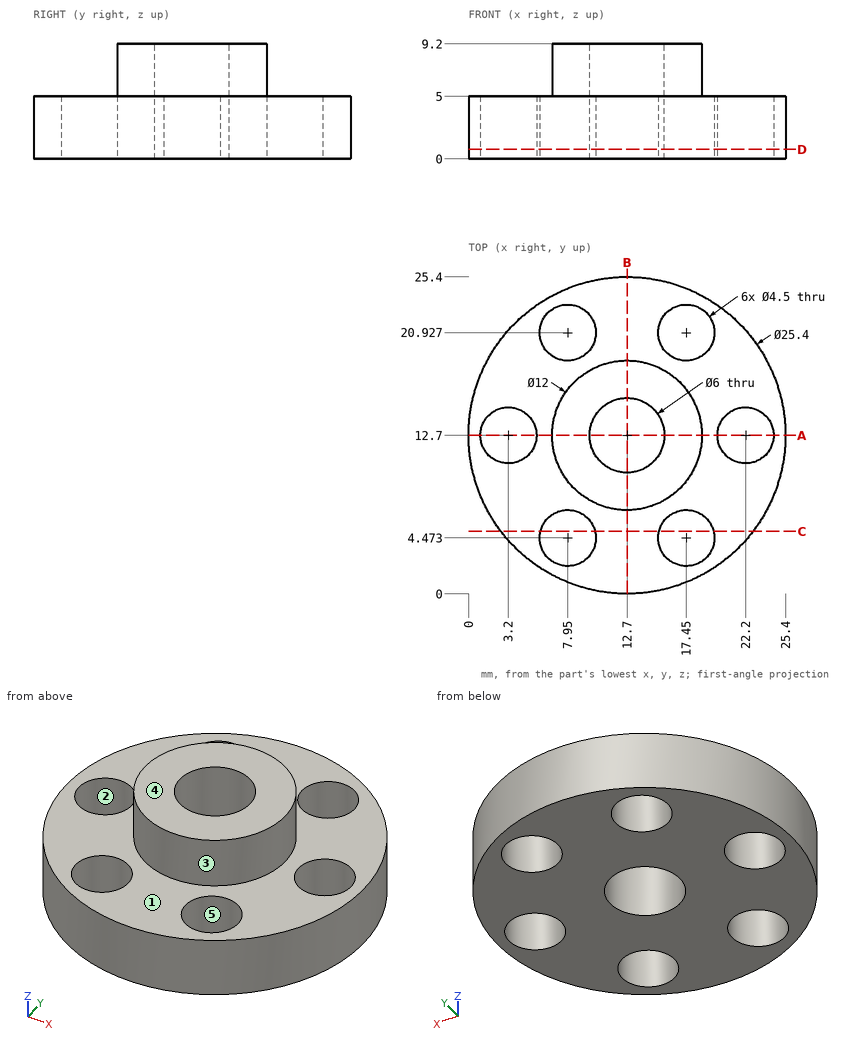
Answer from the drawing. Dimensions are ordinates in mm from the lowest x, y and z of the part. A direction names the side the tool comes from. Coordinates: 2 decimals unless noted, no trailing zeros. Order: outer loops, then holes, each group sorted by start corner. A loop starts at its lowest first (then second) coordinate and runs counter-clockwise, first axis right, second up. Notation, with made-up numbers: (26.5, -20.75) - (44.5, -20.75) arc R11 ccw to (44.5, -4.75) - close; hole circle Ø4 at (-32.75, 7.25). An arc over 180 degrees is marked (long way). Put each result on its own line as item: value. Start each with the question number.
1) For the marked faces 1 and 2, determine the directions among +Z, -Z, +X, -X, +Y, -Y from which every point of the face is accessible in a straight line to the end or side of a thin tool.
2) For a pull along X with two mould halves and no side action, classify the marked faces 3, 4 and 5 as released by +X, released by -X, zero draft, split by the parting line, or undercut.
3) Find section D-D (z = 0.75). Give the vertices of the cut face in (x, y), plus the area to 3 significant figures.
4) Flat-ended cylindrical pins translate along their axes: pin 1 (4 mm diameter, centred on x = 3.5, z = 1.5, fed in from +Y); pin 2 (2 mm diameter, centred on x = 9, z = 7.5, fed in from +Y); pin 3 (1 mm diameter, centred on x = 3.5, z = 1, fed in from +Y). Find the tip coordinate at first contact, or state that the pin passes through.
5) Find section B-B (x = 12.7). Give the vertices of the cut face in (y, z), plus the area to 3 significant figures.
6) Find section C-C (y = 5). Give the vertices of the cut face in (x, z).
7) Find section A-A (y = 12.7). Give the vertices of the cut face in (x, z).
8) Find the intervals of material crossed by line 1 (Y direction, x = 7.95, z = 3.3); line 2 (Y direction, x = 17.75, z = 2.5); line 3 (Y direction, x = 12.7, z = 5.5), in increasing order. Write a range as from..to.
Results list:
1. face 1: +Z
1. face 2: +Z, -Z
2. face 3: split by the parting line
2. face 4: zero draft
2. face 5: undercut
3. outline: circle Ø25.4 at (12.7, 12.7); hole circle Ø4.5 at (3.2, 12.7); hole circle Ø4.5 at (7.95, 4.47); hole circle Ø4.5 at (7.95, 20.93); hole circle Ø6 at (12.7, 12.7); hole circle Ø4.5 at (17.45, 4.47); hole circle Ø4.5 at (17.45, 20.93); hole circle Ø4.5 at (22.2, 12.7)
3. area: 383 mm^2
4. pin 1: stops at y = 23.16
4. pin 2: stops at y = 18.06
4. pin 3: stops at y = 21.95
5. outline: (0, 0) - (9.7, 0) - (9.7, 9.2) - (6.7, 9.2) - (6.7, 5) - (0, 5) - close; (15.7, 0) - (25.4, 0) - (25.4, 5) - (18.7, 5) - (18.7, 9.2) - (15.7, 9.2) - close
5. area: 122 mm^2
6. outline: (2.6, 0) - (5.76, 0) - (5.76, 5) - (2.6, 5) - close; (10.14, 0) - (15.26, 0) - (15.26, 5) - (10.14, 5) - close; (19.64, 0) - (22.8, 0) - (22.8, 5) - (19.64, 5) - close
7. outline: (0, 0) - (0.95, 0) - (0.95, 5) - (0, 5) - close; (5.45, 0) - (9.7, 0) - (9.7, 9.2) - (6.7, 9.2) - (6.7, 5) - (5.45, 5) - close; (15.7, 0) - (19.95, 0) - (19.95, 5) - (18.7, 5) - (18.7, 9.2) - (15.7, 9.2) - close; (24.45, 0) - (25.4, 0) - (25.4, 5) - (24.45, 5) - close
8. line 1: y = 0.92..2.22, 6.72..18.68, 23.18..24.48
8. line 2: y = 1.05..2.24, 6.7..18.7, 23.16..24.35
8. line 3: y = 6.7..9.7, 15.7..18.7
